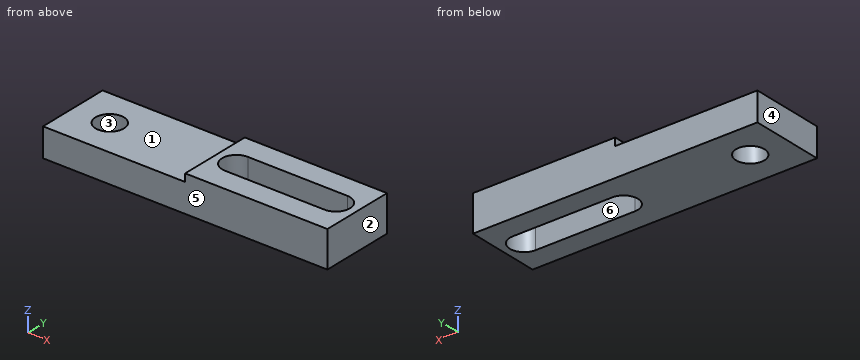
from build123d import *

# Parameters (mm, degrees)
F1_DEPTH = 20
F3_DEPTH = 25.4
F4_DEPTH = 25.4
F5_W     = 100
F5_H     = 52
F6_DEPTH = 20
F8_DEPTH = 25.4
F9_DEPTH = 25.4


with BuildPart() as f1:
    # F0 (on Top) → F1 (new body)
    with BuildSketch(Plane.XY):
        with BuildLine():
            Line((0, 26), (0, 0))
            Line((0, 0), (100, 0))
            Line((100, 0), (100, 26))
            Line((100, 26), (95, 26))
            ThreePointArc((95, 26), (92.0710678119, 18.9289321881), (85, 16))
            Line((85, 16), (15, 16))
            ThreePointArc((15, 16), (7.9289321881, 18.9289321881), (5, 26))
            Line((5, 26), (0, 26))
        make_face()
    extrude(amount=F1_DEPTH)

    # F2 (on face) → F3 (cut)
    with BuildSketch(Plane.XY.offset(20)):
        Polygon((85.6833907061, 35.9766215295), (15.6840754541, 35.9765746012), (15.6840754541, 16.0234253988), (85.6833907061, 16.0233784705), align=None)
    extrude(amount=-F3_DEPTH, mode=Mode.SUBTRACT)

    # F2 (on face) → F4 (cut)
    with BuildSketch(Plane.XY.offset(20)):
        Polygon((85.6833907061, 35.9766215295), (15.6840754541, 35.9765746012), (15.6840754541, 16.0234253988), (85.6833907061, 16.0233784705), align=None)
    extrude(amount=-F4_DEPTH, mode=Mode.SUBTRACT)

    # F5 (on Top) → F6 (join)
    with BuildSketch(Plane.XY):
        with Locations((-50, 26)):
            Rectangle(F5_W, F5_H)
    extrude(amount=F6_DEPTH)

    # F7 (on face) → F8 (cut)
    with BuildSketch(Plane.XY.offset(20)):
        with BuildLine():
            ThreePointArc((-84, 26), (-74, 16), (-64, 26))
            ThreePointArc((-64, 26), (-74, 36), (-84, 26))
        make_face()
    extrude(amount=-F8_DEPTH, mode=Mode.SUBTRACT)

    # F0 (on Top) → F9 (join)
    with BuildSketch(Plane.XY):
        with BuildLine():
            Line((0, 26), (0, 0))
            Line((0, 0), (100, 0))
            Line((100, 0), (100, 26))
            Line((100, 26), (95, 26))
            ThreePointArc((95, 26), (92.0710678119, 18.9289321881), (85, 16))
            Line((85, 16), (15, 16))
            ThreePointArc((15, 16), (7.9289321881, 18.9289321881), (5, 26))
            Line((5, 26), (0, 26))
        make_face()
        with BuildLine():
            Line((0, 52), (0, 26))
            Line((0, 26), (5, 26))
            ThreePointArc((5, 26), (7.9221367888, 33.0642658758), (14.9807704728, 35.9999815112))
            Line((14.9807704728, 35.9999815112), (84.9876315002, 35.999992351))
            ThreePointArc((84.9876315002, 35.999992351), (92.0666935338, 33.0754393856), (95, 26))
            Line((95, 26), (100, 26))
            Line((100, 26), (100, 52))
            Line((100, 52), (0, 52))
        make_face()
    extrude(amount=F9_DEPTH)


solid = f1.part
Source: CAD feature listing. Evaluate the final solid. Frame: model axes, mm. Face numbers are marked on the shaded views. A direction names the side the tool comes from. Round coordinates to 2 decimals unless told otherwise and drop trailing zeros. Loops run counter-clockwise (first coordinate to the right, second up) from the corner with the lowest first, then second, coordinate; pieces in that order, holes last. Notation, with made-up numbers: M 67,1.5 L 112,1.5 A21 cw 112,14.5 Z; hole C 32,-27.75 d6. An arc over 180 degrees is marked long. Return JSON: item names as keys, results as strings. Group by question number.
1. Section query C-C on y = 18.5. Output: boundary loops of the cut face in (x, z), and give its area (3 significant figures).
2. Pin query (flat end, axial travel): pin 1 (15.5 mm diameter, centred on x = -57.5, y = 28.5, fed in from +Z); pin 2 (18 mm diameter, centred on x = -74, y = 26, fed in from +Z); pin 3 (2.5 mm diameter, centred on y = 28.5, z = 22.5, fed in from -X). Return the tip coordinate at first contact, or that it passes through.
3. Section query A-A on x = 35.5. Output: boundary loops of the cut face in (y, z), and give its area (3 significant figures).
4. Material intervals for line 1 along Y through (x, z) = (16, 2); line 2 along X through (y, z) = (28, 2.5); line 3 along X through (y, z) = (30.5, 14.5), sorted ascending. Write a range as from..to.
5. Section query B-B on z = 8. Output: boundary loops of the cut face in (x, y), and give its area (3 significant figures).
6. Section query D-D on y = 40.5. Output: boundary loops of the cut face in (x, z), and give its area (3 significant figures).
7. Mould query, pull axis X, two halves, no side actions, for the marked faces 1, 2, 3 and 4. Classes: released by +X, released by -X, zero draft, split by the parting line, or undercut.
8. Reachability of the marked faces 5 and 6 from +Z, -Z, +X, -X, +Y, -Y: full face, straight path, thin tool, end or side. Return the list, or none.
Checks:
{
 "1": {"outline": "M -100,0 L -80.61,0 L -80.61,20 L -100,20 Z; M -67.39,0 L 8.39,0 L 8.39,25.4 L 0,25.4 L 0,20 L -67.39,20 Z; M 91.61,0 L 100,0 L 100,25.4 L 91.61,25.4 Z", "area": "2,160 mm²"},
 "2": {"pin 1": "stops at z = 20", "pin 2": "passes through", "pin 3": "stops at x = 0"},
 "3": {"outline": "M 0,0 L 16,0 L 16,25.4 L 0,25.4 Z; M 36,0 L 52,0 L 52,25.4 L 36,25.4 Z", "area": "813 mm²"},
 "4": {"line 1": "y = 0..16, 36..52", "line 2": "x = -100..-83.8, -64.2..5.2, 94.8..100", "line 3": "x = -100..-82.93, -65.07..6.07, 93.93..100"},
 "5": {"outline": "M -100,0 L 100,0 L 100,52 L -100,52 Z; hole C -74,26 d20; hole M 14.98,36 A10 ccw 15,16 L 85,16 A10 ccw 84.99,36 Z", "area": "8,370 mm²"},
 "6": {"outline": "M -100,0 L 100,0 L 100,25.4 L 0,25.4 L 0,20 L -100,20 Z", "area": "4,540 mm²"},
 "7": {"face 1": "zero draft", "face 2": "released by +X", "face 3": "undercut", "face 4": "released by -X"},
 "8": {"face 5": "+Z, -Z, +X, -X, -Y", "face 6": "+Z, -Z"}
}
